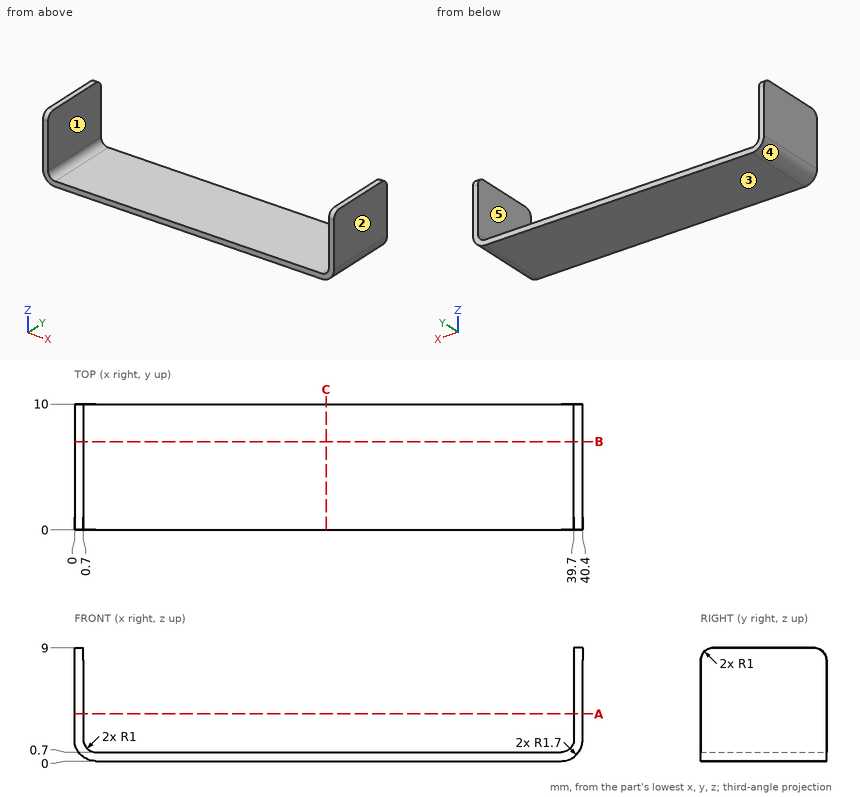
Job drawing, mm, ordinate dimensions from the low corner. One solid piece. A direction names the side the tool comes from. Give positions to 0.01 mm unless a question says otherwise; leave off trailing zeros. Order: outer loops, then holes, each group sorted by start corner. A loop starts at its lowest first (then second) coordinate and runs counter-clockwise, first axis right, second up. Notation, with made-up numbers: (54.5, -7.75) - (94.5, -7.75) arc R15 cw to (94.5, 18.25) - close; hole circle Ø2 at (38, -20.5). An arc over 180 degrees is marked (long way). One line per question, with ' | ' between items.
1. Band-saw the part on C-C on x = 20. List the corners of the cut face in (y, z).
Filled in:
outline: (0, 0) - (10, 0) - (10, 0.7) - (0, 0.7) - close
2. Drill centre lines: probe 1 along X at (y, z) = (5, 4.5); probe 2 along Z at (x, y) = (26.5, 7). Where is each one in solid material? Low to high.
Filled in:
probe 1: 0 to 0.7, 39.7 to 40.4 | probe 2: 0 to 0.7
3. Band-saw the part on A-A on z = 3.75. List the corners of the cut face in (x, y).
Filled in:
outline: (0, 0) - (0.7, 0) - (0.7, 10) - (0, 10) - close; (39.7, 0) - (40.4, 0) - (40.4, 10) - (39.7, 10) - close
4. Drop a flat-ended pin along its axis: P1, Ø1.5, axis at x = 22, y = 3, coming from the +Z side. Give the stop position or say it passes through.
Filled in:
P1: z = 0.7
5. Pull direction X, two halves, no side cores. Call the marked faces 3, 4 and 5: +X half, -X half, draft (parallel to the pull), parting line (faces both ways), or undercut.
Filled in:
face 3: draft | face 4: -X half | face 5: undercut
6. Band-saw the part on B-B on y = 7. List the corners of the cut face in (x, z), then the cut area to 3 significant figures.
Filled in:
outline: (0, 1.7) arc R1.7 ccw to (1.7, 0) - (38.7, 0) arc R1.7 ccw to (40.4, 1.7) - (40.4, 9) - (39.7, 9) - (39.7, 1.7) arc R1 cw to (38.7, 0.7) - (1.7, 0.7) arc R1 cw to (0.7, 1.7) - (0.7, 9) - (0, 9) - close | area: 39.1 mm²
7. Which spindle directions (+Z, -Z, +X, -X, +Y, -Y) get a long thin tool onto all of the face, cutting with end or side? Do the marked faces 1 and 2. Say none if no direction does.
Filled in:
face 1: +Z, +Y, -Y | face 2: +Z, -Z, +X, +Y, -Y
